Work out the finished part from the listing and answer in its coordinate system (mm). A direction names the side the tool comes from. Round coordinates to 2 decimals unless told otherwise and drop trailing zeros. Write each loop counter-clockwise with the first axis right and the second up, starting at its lowest first coordinate (ties: lowest second). Pieces come first, ordered by that corner, then holes.
1. A tool of negligible diameter and unlimited length cuts with its end or side. For faces 1 (the face through (4, 4, 2)), 2 (the face through (0, 8, 12)), 3 (the face through (0, 8, 2.5)), 4 (the face through (8, 0, 2.5)), 5 (the face through (-9, 0, 2.5)), from which of +Z, -Z, +X, -X, +Y, -Y can it reach the whole face along a straight path? Write none if from no direction.
2. Flat-ended cylindrical pins translate along their axes: pin 1 Ø3 at (x, z) = (6.5, 3.5) entering from +Y; pin 2 Ø8 at (x, z) = (2, 12.5) entering from -Y; pin 3 Ø2.5 at (x, y) = (-4.24, -4.24) entering from +Z; pin 4 Ø8 at (y, z) = (3, 16.5) entering from -X. Find the tip coordinate at first contact, or state that the pin passes through.
3. Find section A-A (z = 15.5). Write down the section's boundary in (x, y).
4. Straight lines are drawn through the part: probe 1 along Z at (x, y) = (-9.25, -3.5); probe 2 along Z at (x, y) = (4, 2.75); probe 3 along X at (y, z) = (7.75, 0.75). For each, find the intervals that lie inside material, in ascending order.
5. Determine the mould class of faces 6 (the face through (0, -9, 12)), 7 (the face through (6, -6, 2)), 8 (the face through (-0.54, 2.44, 19.63)) for opening direction Y: pulls with the +Y half, pulls with the -Y half, needs draft (parallel to the pull), parting line crosses it, or undercut.
6. Find section B-B (z = 9.75). Write down the section's boundary in (x, y).
Autodesk Fusion 360 part; units mm, degrees
sketch "Sketch1" plane through (0, 0, 0) normal (0, 0, 1) x (1, 0, 0)
  circle A0 centre (0, 0) radius 2.5
  circle A1 centre (0, 0) radius 11.5
  line L0 (-5.6569, 5.6569) -> (5.6569, -5.6569) construction
  line L1 (4.2426, 4.2426) -> (-4.2426, -4.2426) construction
  circle A2 centre (-5.6569, 5.6569) radius 1
  circle A3 centre (4.2426, 4.2426) radius 1
  circle A4 centre (5.6569, -5.6569) radius 1
  circle A5 centre (-4.2426, -4.2426) radius 1
  line L2 (0, 0) -> (4, 0) construction
  circle A6 centre (0, 0) radius 1
  dimension "d1" = 5
  dimension "d2" = 23
  dimension "d3" = 12
  dimension "d4" = 16
  dimension "d5" = 2
  dimension "d6" = 45
  dimension "d7" = 2
extrude "Extrude1" add sketch "Sketch1" against normal blind 2 contours A6
extrude "Extrude2" add sketch "Sketch1" along normal blind 14.7 contours A0 | A1 | A2 | A3 | A4 | A5 | A6
extrude "Extrude3" add sketch "Sketch1" against normal blind 0.2 contours A0
extrude "Extrude4" cut sketch "Sketch1" along normal blind 2 contours A2 | A3 | A4 | A5
extrude "Extrude5" add sketch "Sketch1" along normal blind 24.7 contours A0 | A6
fillet "Fillet1" radius 1 1 edges at (-10.7218, -4.1586, 0)
chamfer "Chamfer1" distance 4 distance2 2 1 edges at (-10.7218, -4.1586, 14.7) measured on face at (8.4479, -0.6955, 14.7)
sketch "Sketch2" plane through (0, 0, 0) normal (0, 0, -1) x (1, 0, 0)
  circle A0 centre (0, 0) radius 2.5
  circle A1 centre (4.2426, -4.2426) radius 1
  circle A2 centre (-5.6569, -5.6569) radius 1
  circle A3 centre (5.6569, 5.6569) radius 1
  circle A4 centre (-4.2426, 4.2426) radius 1
  circle A5 centre (0, 0) radius 10.5
  spline S0 degree 2 poles (-4.4476, 10.6051) (0, 0) (4.4476, 10.6051) knots 0 0 0 1.552673 1.552673 1.552673 weights 1 1.5 1
  spline S1 degree 2 poles (-10.6051, -4.4476) (0, 0) (-10.6051, 4.4476) knots 0 0 0 1.552673 1.552673 1.552673 weights 1 1.5 1
  spline S2 degree 2 poles (4.4476, -10.6051) (0, 0) (-4.4476, -10.6051) knots 0 0 0 1.552673 1.552673 1.552673 weights 1 1.5 1
  spline S3 degree 2 poles (10.6051, 4.4476) (0, 0) (10.6051, -4.4476) knots 0 0 0 1.552673 1.552673 1.552673 weights 1 1.5 1
  circle A6 centre (0, 0) radius 11.5
  line L0 (-4.4476, 10.6051) -> (4.4476, 10.6051) construction
  dimension "d24" = 360
extrude "Extrude6" cut sketch "Sketch2" against normal blind 2.5 contours A5 S3 | A5 S3 A6 | A5 S0 | A5 S0 A6 | A5 S2 A6 | A5 S2 | A5 S1 | A5 S1 A6
extrude "Extrude7" cut sketch "Sketch2" along normal blind -14.7 and the other way blind 12 contours A5 S3 | A5 S3 A6 | A5 S0 | A5 S0 A6 | A5 S2 A6 | A5 S2 | A5 S1 | A5 S1 A6
Worked answers:
1. face 1: -Z
1. face 2: +Z, +Y
1. face 3: -Z, +Y
1. face 4: -Z, +X
1. face 5: -Z, -X
2. pin 1: stops at y = 10.36
2. pin 2: stops at y = -11.5
2. pin 3: stops at z = 14.7
2. pin 4: stops at x = -10.5
3. outline: circle Ø5 at (0, 0)
4. probe 1: z = 2.5 to 12
4. probe 2: z = 0 to 14.7
4. probe 3: x = -8.45 to -3.15, 3.15 to 8.45
5. face 6: needs draft
5. face 7: undercut
5. face 8: parting line crosses it
6. outline: circle Ø23 at (0, 0)
